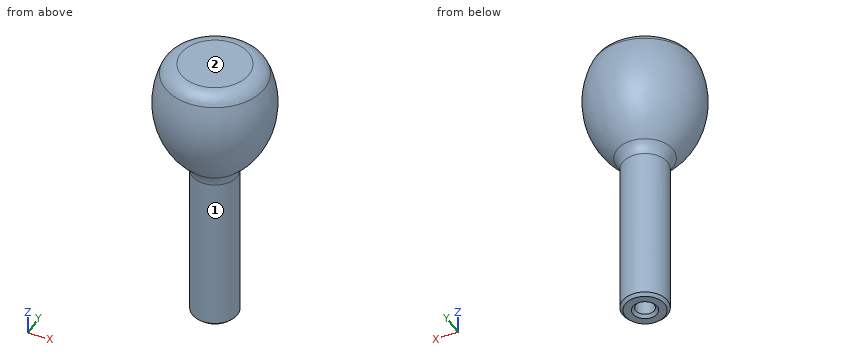
```python
from build123d import *

# Parameters (mm, degrees)
F2_R     = 3
F3_R     = 1.65
F4_DEPTH = 20
F5_SIZE  = 0.5


with BuildPart() as f1:
    # F0 (on Front) → F1 (revolve)
    with BuildSketch(Plane.XZ):
        with BuildLine():
            Line((0, 50), (0, 0))
            Line((0, 0), (4, 0))
            Line((4, 0), (4, 30))
            ThreePointArc((4, 30), (9.718003, 39.267051), (7.880182, 50))
            Line((7.880182, 50), (0, 50))
        make_face()
    revolve(axis=Axis((0, 0, 42.201201), (0, 0, -1)))

    # F2
    f2_edges = [f1.edges().sort_by_distance(p)[0] for p in [
        (-7.880182, 0, 50),
        (-4, 0, 30),
    ]]
    fillet(f2_edges, radius=F2_R)

    # F3 (on face) → F4 (cut)
    with BuildSketch(Plane(origin=(0, 0, 0), x_dir=(1, 0, 0), z_dir=(0, 0, -1))):
        Circle(F3_R)
    extrude(amount=-F4_DEPTH, mode=Mode.SUBTRACT)

    # F5
    f5_edges = [f1.edges().sort_by_distance(p)[0] for p in [
        (-1.65, 0, 0),
        (-4, 0, 0),
    ]]
    chamfer(f5_edges, length=F5_SIZE)


solid = f1.part
```
Can you work these out from the model? Positions are in its coordinate system, mm. Face numbers are marked on the shaded views. A direction names the side the tool comes from. Round coordinates to 2 decimals unless told otherwise and drop trailing zeros. Loops run counter-clockwise (first coordinate to the right, second up) from the corner with the lowest first, then second, coordinate; pieces in that order, holes last.
Item 1: Please list where these lines run through material, in increasing order: L1, parallel to Y at x = 0, z = 13.75; L2, parallel to X at y = -1.25, z = 8.
Item 2: Which directions (+Z, -Z, +X, -X, +Y, -Y) give clear straight access to the entire face, cutting with the end or side of a thin tool? Please do the marked faces 1 and 2.
Item 3: Suppose I cut it at A-A, the plane z = 21.5. Write out the boundary of the cut face in (x, y).
Item 4: Will these pins go through, and if not, where does the flat tip stop? pin 1 Ø5 at (x, y) = (7, 4) entering from -Z; pin 2 Ø6 at (y, z) = (-4, 36) entering from -X; pin 3 Ø4 at (x, y) = (-4.5, -5.5) entering from -Z; pin 4 Ø3 at (y, z) = (-6, 6) entering from -X.
Reported:
1. L1: y = -4 to -1.65, 1.65 to 4
1. L2: x = -3.8 to -1.08, 1.08 to 3.8
2. face 1: -Z
2. face 2: +Z, +X, -X, +Y, -Y
3. outline: circle Ø8 at (0, 0)
4. pin 1: stops at z = 31.38
4. pin 2: stops at x = -9.27
4. pin 3: stops at z = 30.94
4. pin 4: passes through
